Can you work these out from the model? Positions are in its coordinate system, mm. Face numbers are marked on the shaded views. Coordinates: 2 decimals unless noted, no trailing zeros. Loops run counter-clockwise (first coordinate to the right, second up) from the corner with the lowest first, then second, coordinate; pieces in that order, holes last. Notation, with made-up numbers: M -32.75,78.5 L -9.75,78.5 A18 ccw -9.75,110.5 Z; hole C 83,-6.5 d5. An arc over 180 degrees is marked long. Answer as a JSON object with one key per item and string values. Group by question number.
Item 1: We'd pull the mould along Z, two halves only. Please class the marked faces 1, 2 and 3: +Z half, -Z half, draft (parallel to the pull), parting line (faces both ways), or undercut.
Item 2: Suppose I cut it at C-C (x = 8.5). Write out the boundary of the cut face in (y, z), then the cut area to 3 significant figures.
Item 3: I'm going to push flat-ended pins straight in: pin 1 Ø1 at (x, z) = (40, 3.5) entering from -Y; pin 2 Ø1.5 at (x, y) = (37, 4.5) entering from -Z; pin 3 Ø2 at (x, y) = (42, -1) entering from -Z; pin 4 Ø1.5 at (x, y) = (42.5, 3) entering from +Z. Where does each tip first touch, or does it pass through?
Item 4: If I drill on line 1 (Y direction, x = 64.5, z = 0); line 2 (X direction, y = 3.5, z = 4.5); line 3 (X direction, y = -7.25, z = 2.5), over which ranges is the centre line in solid material (lowest first)?
Item 5: Suppose I cut it at B-B (z = -5.5). Write out the boundary of the cut face in (x, y), then the cut area to 3 significant figures.
Item 6: Suppose I cut it at A-A (y = 2). Write out the boundary of the cut face in (x, z).
```python
from build123d import *

# Parameters (mm, degrees)
SKETCH_1_R          = 9
EXTRUDE_1_DEPTH     = 65
SKETCH_2_R          = 7.5
CUT_EXTRUDE_1_DEPTH = 1
SKETCH_3_R          = 3
EXTRUDE_2_DEPTH     = 1.5


with BuildPart() as part:
    # Эскиз1 → Бобышка-Вытянуть1 (new body)
    with BuildSketch(Plane(origin=(0, 0, 0), x_dir=(0, 0, -1), z_dir=(1, 0, 0))):
        Circle(SKETCH_1_R)
    extrude(amount=EXTRUDE_1_DEPTH)

    # Эскиз2 → Вырез-Вытянуть1 (cut)
    with BuildSketch(Plane(origin=(65, 0, 0), x_dir=(0, 0, -1), z_dir=(1, 0, 0))):
        Circle(SKETCH_2_R)
    extrude(amount=-CUT_EXTRUDE_1_DEPTH, mode=Mode.SUBTRACT)

    # Эскиз3 → Бобышка-Вытянуть2 (add)
    with BuildSketch(Plane(origin=(64, 0, 0), x_dir=(0, 0, -1), z_dir=(1, 0, 0))):
        with Locations((-0.192251795, 0.103684868)):
            Circle(SKETCH_3_R)
    extrude(amount=EXTRUDE_2_DEPTH)


solid = part.part
```
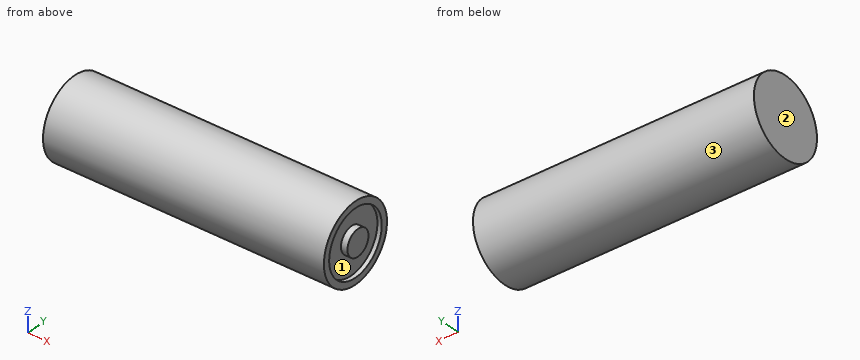
From the geometry:
{
 "1": {"face 1": "undercut", "face 2": "draft", "face 3": "parting line"},
 "2": {"outline": "C 0,0 d18", "area": "254 mm2"},
 "3": {"pin 1": "y = -8.49", "pin 2": "z = -8.18", "pin 3": "z = -9", "pin 4": "z = 8.71"},
 "4": {"line 1": "-9 to -7.5, -2.89 to 3.1, 7.5 to 9", "line 2": "0 to 64", "line 3": "0 to 65"},
 "5": {"outline": "M 0,-7.12 L 65,-7.12 L 65,-5.1 L 64,-5.1 L 64,5.1 L 65,5.1 L 65,7.12 L 0,7.12 Z", "area": "916 mm2"},
 "6": {"outline": "M 0,-8.77 L 65,-8.77 L 65,-7.23 L 64,-7.23 L 64,-2.13 L 65.5,-2.13 L 65.5,2.52 L 64,2.52 L 64,7.23 L 65,7.23 L 65,8.77 L 0,8.77 Z"}
}
